Job drawing, mm, ordinate dimensions from the low corner. One solid piece. A direction names the side the tool comes from. Give positions to 0.01 mm unless a question says otherwise; leave off trailing zeros. Loops run counter-clockwise (first coordinate to the right, second up) from the corner with the lowest first, then second, coordinate; pieces in that order, holes last. Notation, with made-up numbers: M 85,35.5 L 122,35.5 A31 ccw 122,68.5 Z; hole C 84.25,-18.5 d5. An arc over 180 degrees is marked long. Answer in a Markdown table with one row per item.
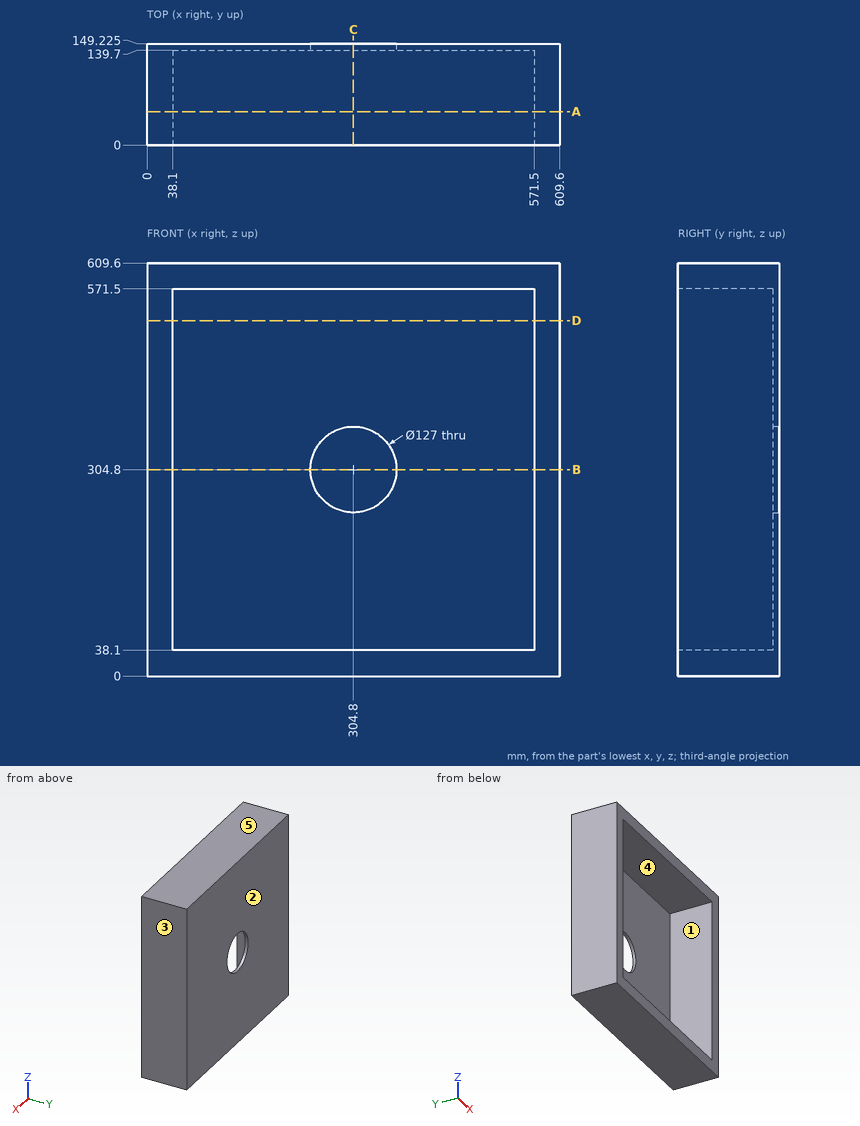
(1) Saw through at D-D (z = 524.5). Write the cut outline in (x, y) (3 decimals), plus the area to 3 significant figures.
Recorded:
| item | result |
|---|---|
| outline | M 0,0 L 38.1,0 L 38.1,139.7 L 571.5,139.7 L 571.5,0 L 609.6,0 L 609.6,149.225 L 0,149.225 Z |
| area | 16,500 mm^2 |
(2) Pull direction X, two halves, no side cores. Call the marked faces 3, 4 and 5: +X half, -X half, draft (parallel to the pull), parting line (faces both ways), or undercut.
Recorded:
| item | result |
|---|---|
| face 3 | +X half |
| face 4 | undercut |
| face 5 | draft |
(3) Saw through at A-A (y = 49.5). Write the cut outline in (x, z), plus the area to 3 significant figures.
Recorded:
| item | result |
|---|---|
| outline | M 0,0 L 609.6,0 L 609.6,609.6 L 0,609.6 Z; hole M 38.1,38.1 L 571.5,38.1 L 571.5,571.5 L 38.1,571.5 Z |
| area | 87,100 mm^2 |
(4) Saw through at C-C (x = 304.8). Write the cut outline in (y, z) (3 decimals).
Recorded:
| item | result |
|---|---|
| outline | M 0,0 L 149.225,0 L 149.225,241.3 L 139.7,241.3 L 139.7,38.1 L 0,38.1 Z; M 0,571.5 L 139.7,571.5 L 139.7,368.3 L 149.225,368.3 L 149.225,609.6 L 0,609.6 Z |
(5) Drill centre lines: line 1 along Z through (x, y) = (566, 130.5); line 2 along X through (y, z) = (143, 304). Where is each one in solid material? Low to high.
Recorded:
| item | result |
|---|---|
| line 1 | z = 0 to 38.1, 571.5 to 609.6 |
| line 2 | x = 0 to 241.31, 368.29 to 609.6 |
(6) Saw through at B-B (z = 304.8). Write the cut outline in (x, y) (3 decimals).
Recorded:
| item | result |
|---|---|
| outline | M 0,0 L 38.1,0 L 38.1,139.7 L 241.3,139.7 L 241.3,149.225 L 0,149.225 Z; M 368.3,139.7 L 571.5,139.7 L 571.5,0 L 609.6,0 L 609.6,149.225 L 368.3,149.225 Z |
(7) Which spindle directions (+Z, -Z, +X, -X, +Y, -Y) get a long thin tool onto all of the face, cutting with end or side? Do the marked faces 1 and 2. Say none if no direction does.
Recorded:
| item | result |
|---|---|
| face 1 | -Y |
| face 2 | +Z, -Z, +X, -X, +Y |
